Part model, mm, in its own coordinate system. A direction names the side the tool comes from. Give positions to 0.01 mm unless a question says otherwise; leave off trailing zeros. Write each loop counter-clockwise with the first axis right and the second up, starting at its lowest first coordinate (ties: lowest second). Pieces come first, ordered by that corner, then holes.
```python
from build123d import *

# Parameters (mm, degrees)
PAD_DEPTH    = 6
SKETCH001_R  = 1.2
POCKET_DEPTH = 50


with BuildPart() as part:
    # Sketch → Pad (new body)
    with BuildSketch(Plane.XY):
        Polygon((-5, 11.7), (5, 11.7), (35, 33.7), (45, 33.7), (45, 30.2), (35, 30.2), (35, 26), (45, 26), (45, 22), (35, 22), (5, 0), (-5, 0), (-5, 4), (5, 4), (5, 7.7), (-5, 7.7), align=None)
        Polygon((9.032025, 10.656818), (30.967975, 26.743182), (30.967975, 23.043182), (9.032025, 6.956818), align=None, mode=Mode.SUBTRACT)
    extrude(amount=PAD_DEPTH)

    # Sketch001 (on Face12 of Pad) → Pocket (cut)
    with BuildSketch(Plane.XZ):
        with Locations((0, 3)):
            Circle(SKETCH001_R)
        with Locations((40, 3)):
            Circle(SKETCH001_R)
    extrude(amount=-POCKET_DEPTH, mode=Mode.SUBTRACT)


solid = part.part
```
1) 3-axis set-ups, long thin cutter, end or side, ignore diameter. For faces 1 (the face through (41, 26, 2)), 2 (the face through (41, 33.7, 2)), 3 (the face through (-1, 11.7, 2)), 4 (the face through (19.85, 18.59, 2.96)), 5 (the face through (-1, 4, 2)): which of +Z, -Z, +X, -X, +Y, -Y reach the whole face in a straight line?
Answers follow:
face 1: +Z, -Z, +X
face 2: +Z, -Z, +X, -X, +Y
face 3: +Z, -Z, -X, +Y
face 4: +Z, -Z
face 5: +Z, -Z, -X
2) Saw through at B-B, the plane z = 4.9. Write the cut outline in (x, y).
Answers follow:
outline: (-5, 0) - (5, 0) - (35, 22) - (45, 22) - (45, 26) - (35, 26) - (35, 30.2) - (45, 30.2) - (45, 33.7) - (35, 33.7) - (5, 11.7) - (-5, 11.7) - (-5, 7.7) - (5, 7.7) - (5, 4) - (-5, 4) - close; hole (9.03, 6.96) - (30.97, 23.04) - (30.97, 26.74) - (9.03, 10.66) - close
3) Pin check, flat tips, straight feed: pin 1 Ø1.8 at (x, z) = (42.5, 2) entering from -Y; pin 2 Ø3 at (y, z) = (24.5, 2.5) entering from -X; pin 3 Ø2 at (y, z) = (27.5, 2) entering from +X. Stop position of each tip, or through.
Answers follow:
pin 1: stops at y = 22
pin 2: stops at x = 20.41
pin 3: stops at x = 35
4) Saw through at C-C, the plane y = 19. Write the cut outline in (x, z).
Answers follow:
outline: (14.95, 0) - (20.41, 0) - (20.41, 6) - (14.95, 6) - close; (25.45, 0) - (30.91, 0) - (30.91, 6) - (25.45, 6) - close
5) Wall check: L1, parallel to Z at x = 40, y = 24.75; L2, parallel to Y at x = 42, z = 1.3; L3, parallel to X at y = 10.5, z = 2.4. Give the ranges that are in metal, low to high.
Answers follow:
L1: z = 0 to 1.8, 4.2 to 6
L2: y = 22 to 26, 30.2 to 33.7
L3: x = -5 to -1.04, 1.04 to 9.03, 13.86 to 19.32
6) Saw through at D-D, the plane y = 10. Write the cut outline in (x, z), then the cut area to 3 significant figures.
Answers follow:
outline: (-5, 0) - (9.03, 0) - (9.03, 6) - (-5, 6) - close; (13.18, 0) - (18.64, 0) - (18.64, 6) - (13.18, 6) - close; hole circle Ø2.4 at (0, 3)
area: 112 mm2
7) Two-plate mould, pull along Z, no slides. Class faces 6 (the face through (0.65, 1.97, 4.01)), 7 (the face through (18, 18, 6)), 8 (the face through (41.11, 23.97, 2.54)), 9 (the face through (30.968, 25, 3)): +Z half, -Z half, draft (parallel to the pull), parting line (faces both ways), or undercut.
Answers follow:
face 6: undercut
face 7: +Z half
face 8: undercut
face 9: draft
8) Saw through at A-A, the plane x = 0. Write the cut outline in (y, z).
Answers follow:
outline: (0, 0) - (4, 0) - (4, 1.8) - (0, 1.8) - close; (0, 4.2) - (4, 4.2) - (4, 6) - (0, 6) - close; (7.7, 0) - (11.7, 0) - (11.7, 1.8) - (7.7, 1.8) - close; (7.7, 4.2) - (11.7, 4.2) - (11.7, 6) - (7.7, 6) - close
